Geometry check sheet. Reference: the model listing, model coordinates, mm. Face numbers are marked on the shaded views. Round coordinates to 2 decimals unless told otherwise and drop trailing zeros. Order: outer loops, then holes, each group sorted by start corner. A loop starts at its lowest first (then second) coordinate and runs counter-clockwise, first axis right, second up.
(1) Cross-section at C-C on z = -15. Enter the section's corners in (x, y), and give its area (3 significant figures).
(2) Gauge pin test, flat ends, axial feed: P1, Ø2, axis at x = -7, z = -38, coming from the -Y side; P2, Ø6, axis at x = -2, y = -3, coming from the +Z side; P3, Ø3, axis at x = 11, y = -2, coming from the +Z side; P4, Ø2.5, axis at x = -15.75, y = -15.75, coming from the -Z side. Record the tip position at first contact, or that the pin passes through.
(3) Cross-section at D-D on x = 10. Enter the section's corners in (y, z).
(4) Cross-section at A-A on y = 0. Enter the section's corners in (x, z), and give its area (3 significant figures).
(5) Draft check along Z on the marked faces 1, 2 and 3. Enter one of: pulls with the +Z half, pulls with the -Z half, needs draft (parallel to the pull), parting line crosses it, or undercut.
(6) Thickness scan on L1, parallel to Y at x = -15.75, z = -2.85; L2, parallel to Y at x = -15, z = -3. Record the ranges inside material, lowest first.
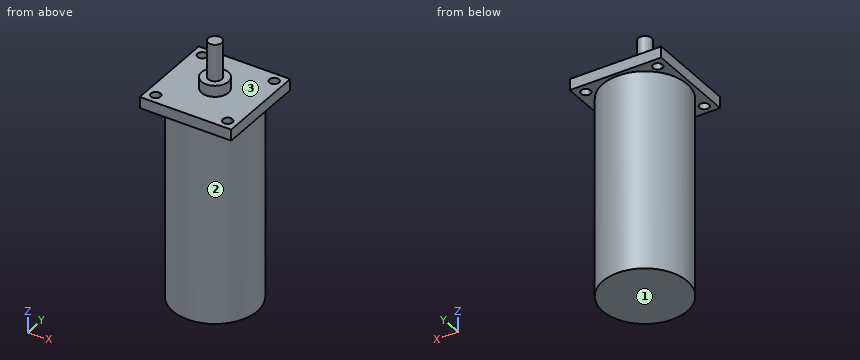
from build123d import *

# Parameters (mm, degrees)
F0_W     = 40
F0_H     = 40
F0_R     = 5.9
F0_R_2   = 2.95
F1_DEPTH = 4.9
F2_DEPTH = 21
F3_DEPTH = 4.9
F4_R     = 18.5
F5_DEPTH = 87


with BuildPart() as f1:
    # F0 (on Top) → F1 (new body)
    with BuildSketch(Plane.XY):
        Rectangle(F0_W, F0_H)
        with BuildLine():
            ThreePointArc((-15.75, 13.65), (-17.2349242405, 17.2349242405), (-13.65, 15.75))
            Line((-13.65, 15.75), (13.65, 15.75))
            ThreePointArc((13.65, 15.75), (15.75, 17.85), (17.85, 15.75))
            ThreePointArc((17.85, 15.75), (17.2349242405, 14.2650757595), (15.75, 13.65))
            Line((15.75, 13.65), (15.75, -13.65))
            ThreePointArc((15.75, -13.65), (17.2349242405, -14.2650757595), (17.85, -15.75))
            ThreePointArc((17.85, -15.75), (15.75, -17.85), (13.65, -15.75))
            Line((13.65, -15.75), (-13.65, -15.75))
            ThreePointArc((-13.65, -15.75), (-17.2349242405, -17.2349242405), (-15.75, -13.65))
            Line((-15.75, -13.65), (-15.75, 13.65))
        make_face(mode=Mode.SUBTRACT)
        with BuildLine():
            Line((13.65, 15.75), (-13.65, 15.75))
            ThreePointArc((-13.65, 15.75), (-14.2650757595, 14.2650757595), (-15.75, 13.65))
            Line((-15.75, 13.65), (-15.75, -13.65))
            ThreePointArc((-15.75, -13.65), (-14.2650757595, -14.2650757595), (-13.65, -15.75))
            Line((-13.65, -15.75), (13.65, -15.75))
            ThreePointArc((13.65, -15.75), (14.2650757595, -14.2650757595), (15.75, -13.65))
            Line((15.75, -13.65), (15.75, 13.65))
            ThreePointArc((15.75, 13.65), (14.2650757595, 14.2650757595), (13.65, 15.75))
        make_face()
        Circle(F0_R, mode=Mode.SUBTRACT)
        Circle(F0_R)
        Circle(F0_R_2, mode=Mode.SUBTRACT)
        Circle(F0_R_2)
    extrude(amount=-F1_DEPTH)

    # F0 (on Top) → F2 (join)
    with BuildSketch(Plane.XY):
        Circle(F0_R_2)
    extrude(amount=F2_DEPTH)

    # F0 (on Top) → F3 (join)
    with BuildSketch(Plane.XY):
        Circle(F0_R)
        Circle(F0_R_2, mode=Mode.SUBTRACT)
    extrude(amount=F3_DEPTH)

    # F4 (on face) → F5 (join)
    with BuildSketch(Plane(origin=(0, 0, -4.9), x_dir=(1, 0, 0), z_dir=(0, 0, -1))):
        Circle(F4_R)
    extrude(amount=F5_DEPTH)


solid = f1.part
Found:
1. outline: circle Ø37 at (0, 0)
1. area: 1,080 mm2
2. P1: stops at y = -17.5
2. P2: stops at z = 21
2. P3: stops at z = 0
2. P4: passes through
3. outline: (-20, -4.9) - (-15.56, -4.9) - (-15.56, -91.9) - (15.56, -91.9) - (15.56, -4.9) - (20, -4.9) - (20, 0) - (-20, 0) - close
4. outline: (-20, -4.9) - (-18.5, -4.9) - (-18.5, -91.9) - (18.5, -91.9) - (18.5, -4.9) - (20, -4.9) - (20, 0) - (5.9, 0) - (5.9, 4.9) - (2.95, 4.9) - (2.95, 21) - (-2.95, 21) - (-2.95, 4.9) - (-5.9, 4.9) - (-5.9, 0) - (-20, 0) - close
4. area: 3,570 mm2
5. face 1: pulls with the -Z half
5. face 2: needs draft
5. face 3: pulls with the +Z half
6. L1: y = -20 to -17.85, -13.65 to 13.65, 17.85 to 20
6. L2: y = -20 to -17.71, -13.79 to 13.79, 17.71 to 20
